from build123d import *

# Parameters (mm, degrees)
F0_W     = 114.3
F0_H     = 25.4
F1_DEPTH = 58.7375
F2_W     = 114.3
F2_H     = 15.875
F3_DEPTH = 31.75
F5_DEPTH = 15.876
F6_R     = 11.90625
F7_DEPTH = 25.401
F9_DEPTH = 58.7385


with BuildPart() as f1:
    # F0 (on Front) → F1 (new body)
    with BuildSketch(Plane.XZ):
        with Locations((4.9286, -44.843187)):
            Rectangle(F0_W, F0_H)
    extrude(amount=-F1_DEPTH)

    # F2 (on face) → F3 (join)
    with BuildSketch(Plane.XY.offset(-32.143187)):
        with Locations((4.9286, 50.8)):
            Rectangle(F2_W, F2_H)
    extrude(amount=F3_DEPTH)

    # F4 (on face) → F5 (cut, through all)
    with BuildSketch(Plane.XZ.offset(-42.8625)):
        Polygon((-52.2214, -0.393187), (-52.2214, -19.443187), (-33.1714, -0.393187), align=None)
        Polygon((62.0786, -0.393187), (43.0286, -0.393187), (62.0786, -19.443187), align=None)
    extrude(amount=-F5_DEPTH, mode=Mode.SUBTRACT)

    # F6 (on face) → F7 (cut, through all)
    with BuildSketch(Plane.XY.offset(-32.143187)):
        with Locations((4.9286, 22.225)):
            Circle(F6_R)
    extrude(amount=-F7_DEPTH, mode=Mode.SUBTRACT)

    # F8 (on face) → F9 (cut, through all)
    with BuildSketch(Plane.XZ):
        Polygon((44.010948, -44.843187), (-34.153748, -44.843187), (-26.8214, -57.543187), (36.6786, -57.543187), align=None)
    extrude(amount=-F9_DEPTH, mode=Mode.SUBTRACT)


solid = f1.part
Verification items for the finished model (mm, model axes). A direction names the side the tool comes from. Coordinates: 2 decimals unless noted, no trailing zeros. Order: outer loops, then holes, each group sorted by start corner. A loop starts at its lowest first (then second) coordinate and runs counter-clockwise, first axis right, second up.
Item 1: Section check A-A, the plane x = -28.5. Enter the section's corners in (y, z).
Filled in:
outline: (0, -57.54) - (58.74, -57.54) - (58.74, -54.64) - (0, -54.64) - close; (0, -44.84) - (58.74, -44.84) - (58.74, -0.39) - (42.86, -0.39) - (42.86, -32.14) - (0, -32.14) - close
Item 2: Material ranges on L1, parallel to Z at x = 23, y = 4.5; L2, parallel to Y at x = -36, z = -19; L3, parallel to Z at x = -35, y = 25, recorded low to high.
Filled in:
L1: z = -44.84 to -32.14
L2: y = 42.86 to 58.74
L3: z = -57.54 to -32.14
Item 3: Access from +Z, -Z, +X, -X, +Y, -Y to the whole of each face (thin tool, end or side, straight path). Record for faces 1 (the face through (-40, 29, -57.543)), 2 (the face through (-30.54, 28.96, -51.1)), 3 (the face through (4, 42.862, -16)).
Filled in:
face 1: -Z, +X, -X, +Y, -Y
face 2: +Y, -Y
face 3: +Z, +X, -X, -Y
Item 4: Release check for a two-part mould opening along X. For faces 4 (the face through (10.42, 11.66, -38.4)), 5 (the face through (4, 58.738, -29)), 6 (the face through (-42.83, 50.69, -10.05)), 7 (the face through (40.293, 28.958, -51.282)) record: +X half, -X half, draft (parallel to the pull), parting line (faces both ways), or undercut.
Filled in:
face 4: undercut
face 5: draft
face 6: -X half
face 7: undercut
Item 5: Section check D-D, the plane z = -43.5. Enter the section's corners in (x, y) (1 decimal).
Filled in:
outline: (-52.2, 0) - (62.1, 0) - (62.1, 58.7) - (-52.2, 58.7) - close; hole circle Ø23.8 at (4.9, 22.2)
Item 6: Section check C-C, the plane y = 51. Enter the section's corners in (x, z).
Filled in:
outline: (-52.22, -57.54) - (-26.82, -57.54) - (-34.15, -44.84) - (44.01, -44.84) - (36.68, -57.54) - (62.08, -57.54) - (62.08, -19.44) - (43.03, -0.39) - (-33.17, -0.39) - (-52.22, -19.44) - close
Item 7: Section check B-B, the plane y = 13. Enter the section's corners in (x, z), then the cut area to 3 significant figures.
Filled in:
outline: (-52.22, -57.54) - (-26.82, -57.54) - (-34.15, -44.84) - (-2.6, -44.84) - (-2.6, -32.14) - (-52.22, -32.14) - close; (12.46, -44.84) - (44.01, -44.84) - (36.68, -57.54) - (62.08, -57.54) - (62.08, -32.14) - (12.46, -32.14) - close
area: 1,810 mm2
Item 8: Depth check by flat-ended pin: pin 1 (17.5 mm diameter, centred on x = 4, y = 22.5, fed in from -Z); pin 2 (4 mm diameter, centred on x = 4, y = 43, fed in from -Z); pin 3 (3 mm diameter, centred on x = -39.5, z = -22.5, fed in from -Y); pin 4 (1.5 mm diameter, centred on x = 23.5, y = 6.5, fed in from +Z). Enter the tip coordinate at first touch or a pass-through.
Filled in:
pin 1: passes through
pin 2: stops at z = -44.84
pin 3: stops at y = 42.86
pin 4: stops at z = -32.14
